from build123d import *

# Parameters (mm, degrees)
SKETCH2_W           = 170
SKETCH2_H           = 82
BOSS_EXTRUDE1_DEPTH = 15
SKETCH6_R           = 2
SKETCH7_W           = 56.062084811
SKETCH7_H           = 3
CUT_EXTRUDE2_DEPTH  = 96.636028792
LPATTERN1_COUNT     = 2
LPATTERN1_PITCH     = 10


with BuildPart() as part:
    # Sketch2 → Boss-Extrude1 (new body)
    with BuildSketch(Plane.XY):
        Rectangle(SKETCH2_W, SKETCH2_H)
    extrude(amount=BOSS_EXTRUDE1_DEPTH)

    # Sweep1: sweep along a path in Sketch5
    with BuildLine(Plane(origin=(0, 0, 0), x_dir=(0, 0, -1), z_dir=(1, 0, 0))) as sweep1_path:
        Line((0, 29.163871958), (5.5, 29.163871958))
        ThreePointArc((5.5, 29.163871958), (11.156854249, 26.820726208), (13.5, 21.163871958))
        Line((13.5, 21.163871958), (13.5, -15.836128042))
    # Sketch6 → Sweep1 (sweep)
    with BuildSketch(Plane(origin=(0, 0, 0), x_dir=(-1, 0, 0), z_dir=(0, 0, -1))):
        with Locations((0, 29.163871958)):
            Circle(SKETCH6_R)
    sweep1 = sweep(path=sweep1_path.line)

    # Sketch7 → Cut-Extrude2 (cut, through all)
    with BuildSketch(Plane(origin=(0, 0, 0), x_dir=(-1, 0, 0), z_dir=(0, 0, -1))):
        with Locations((20.655822978, -30.33067124)):
            Rectangle(SKETCH7_W, SKETCH7_H)
    extrude(amount=-CUT_EXTRUDE2_DEPTH, mode=Mode.SUBTRACT)

    # LPattern1: Sweep1 ×2
    with Locations(*[(-i * LPATTERN1_PITCH, 0, 0) for i in range(1, LPATTERN1_COUNT)]):
        add(sweep1)


solid = part.part
Design review of the part built by this model. Coordinates are the model's own, in mm. A direction names the side the tool comes from. Round coordinates to 2 decimals unless told otherwise and drop trailing zeros. Order: outer loops, then holes, each group sorted by start corner. A loop starts at its lowest first (then second) coordinate and runs counter-clockwise, first axis right, second up.
1) Draft analysis for pull direction Y (two halves, no side actions). For faces 1 (the cylindrical face through (0.43, 27.21, -2.79)), 2 (the flat face through (-1, -41, 7)), 3 (the flat face through (-20, -28.831, 7)), state which applies: released by +Y, released by -Y, zero draft, split by the parting line, or undercut.
The answers:
face 1: split by the parting line
face 2: released by -Y
face 3: undercut
2) Consider section B-B (y = -9.5). State the section outline as (x, z) points, plus the area to 3 significant figures.
The answers:
outline: (-85, 0) - (85, 0) - (85, 15) - (-85, 15) - close; circle Ø4 at (-10, -13.5); circle Ø4 at (0, -13.5)
area: 2,580 mm2
3) Consider section C-C (y = -24). State the section outline as (x, z) points, plus the area to 3 significant figures.
The answers:
outline: (-85, 0) - (85, 0) - (85, 15) - (-85, 15) - close
area: 2,550 mm2
4) Consider section D-D (x = 25.5). State the section outline as (y, z) points.
The answers:
outline: (-41, 0) - (41, 0) - (41, 15) - (-41, 15) - close
5) Machinability: for faces 4 (the flat face through (-1, 41, 7)), 5 (the cylindrical face through (-9.57, 27.21, -2.79)), 6 (the cylindrical face through (0.26, 2.405, -15.483)), 7 (the flat face through (0, -15.836, -13)), 8 (the flat face through (-48.687, -30, 7)), which of the approach directions +Z, -Z, +X, -X, +Y, -Y give a long, thin tool a straight path to every point of the face, cutting with its end or side? Answer none if there is none.
The answers:
face 4: +Z, -Z, +X, -X, +Y
face 5: none
face 6: -Y
face 7: -Z, +X, -X, -Y
face 8: +Z, -Z
6) Clearance check with flat-ended pins moving along their axes: pin 1 Ø3 at (x, z) = (-9.5, -12.5) entering from -Y; pin 2 Ø5 at (y, z) = (31, -6) entering from +X; pin 3 Ø2 at (x, y) = (-67, 10.5) entering from -Z. State where each tip first meets the part, or that it passes through.
The answers:
pin 1: stops at y = -15.84
pin 2: stops at x = 2
pin 3: stops at z = 0
7) For L1, parallel to Z at x = -28, y = -7; L2, parallel to Z at x = -1, y = 18; L3, parallel to X at y = 27, z = -10, list the stretches that pass through material, from the lowest coordinate up.
The answers:
L1: z = 0 to 15
L2: z = -15.23 to -11.77, 0 to 15
L3: x = -11.9 to -8.1, -1.9 to 1.9
8) Consider section A-A (x = -10). State the section outline as (y, z) points, plus the area to 3 significant figures.
The answers:
outline: (-41, 0) - (-31.83, 0) - (-31.83, 15) - (-41, 15) - close; (-28.83, 0) - (27.16, 0) - (27.16, -5.5) arc R6 cw to (21.16, -11.5) - (-15.84, -11.5) - (-15.84, -15.5) - (21.16, -15.5) arc R10 ccw to (31.16, -5.5) - (31.16, 0) - (41, 0) - (41, 15) - (-28.83, 15) - close
area: 1,410 mm2
